Source: CAD feature listing. Evaluate the final solid. Frame: model axes, mm. A direction names the side the tool comes from. Coordinates: 2 decimals unless noted, no trailing zeros. Write each loop counter-clockwise with the first axis right and the second up, starting at its lowest first coordinate (ties: lowest second). Pieces come first, ordered by that corner, then holes. Notation, with made-up numbers: M -33.5,-38.5 L -9.5,-38.5 A20 cw -9.5,-29.5 Z; hole C 50.5,88.5 d4. An arc over 180 degrees is marked long. One line per item, written item: value. Start each with the question number.
Item 1: Cut plane D-D, the plane y = 1.4. Output: boundary loops of the cut face in (x, z) (3 decimals), then the cut area to 3 significant figures.
Item 2: Mould query, pull axis Z, two halves, no side actions, for faces 1 (the cylindrical face through (10.301, 1.521, -5.315)), 2 (the flat face through (10, 1, -15.6)), 3 (the cylindrical face through (6.031, 1.479, 1.176)). Classes: released by +Z, released by -Z, zero draft, split by the parting line, or undercut.
Item 3: Set-up query: faces 4 (the flat face through (15, 1, -5.6)), 5 (the cylindrical face through (5.067, 1.479, -12.124)). Return all of +Z, -Z, +X, -X, +Y, -Y with unobstructed straight access to the full face (end or side cutting, diameter ignored); none if empty.
Item 4: Cut plane A-A, the plane z = 2.3. Output: boundary loops of the cut face in (x, y) (3 decimals), then the cut area to 4 significant figures.
Item 5: Cut plane C-C, the plane z = -10.6. Output: boundary loops of the cut face in (x, y) (3 decimals).
Item 6: Pin query (flat end, axial travel): P1, Ø2.5, axis at x = 5, z = -10.6, coming from the -Y side; P2, Ø1.5, axis at y = 2, z = 0, coming from the +X side; P3, Ø0.9, axis at x = 15.5, y = 1, coming from the +Z side. Return the tip coordinate at first contact, or that it passes through.
Item 7: Ray query, L1, parallel to X at y = 2.3, z = -10.6 (3 decimals); L2, parallel to Z at x = 3.75, y = 1.35; L3, parallel to Z at x = 16.75, y = 0.4. Return the intervals inside material, ascending. Write a range as from..to.
Item 8: Cut plane B-B, the plane x = 5. Output: boundary loops of the cut face in (y, z) (3 decimals), then the cut area to 4 significant figures.
```python
from build123d import *

# Parameters (mm, degrees)
SKETCH1_R           = 1.525
BOSS_EXTRUDE1_DEPTH = 3
FILLET1_R           = 1


with BuildPart() as part:
    # Sketch1 → Boss-Extrude1 (new body)
    with BuildSketch(Plane(origin=(0, 0, 0), x_dir=(1, 0, 0), z_dir=(0, 1, 0))):
        Polygon((10, 5.6), (20, 5.6), (20, 15.6), (0, 15.6), (0, 0), (0, -22.6), (10, -22.6), align=None)
        with Locations(Location((5, 10.6, 0), (0, 0, 270))):
            Circle(SKETCH1_R, mode=Mode.SUBTRACT)
        with Locations(Location((15, 10.6, 0), (0, 0, 270))):
            Circle(SKETCH1_R, mode=Mode.SUBTRACT)
        with Locations(Location((5, -2.3, 0), (0, 0, 270))):
            Circle(SKETCH1_R, mode=Mode.SUBTRACT)
        with Locations(Location((5, -20.3, 0), (0, 0, 270))):
            Circle(SKETCH1_R, mode=Mode.SUBTRACT)
    extrude(amount=BOSS_EXTRUDE1_DEPTH)

    # Fillet1
    fillet1_edges = [part.edges().sort_by_distance(p)[0] for p in [
        (10, 1.5, 22.6),
        (0, 1.5, 22.6),
        (0, 1.5, -15.6),
        (20, 1.5, -15.6),
        (20, 1.5, -5.6),
        (10, 1.5, -5.6),
    ]]
    fillet(fillet1_edges, radius=FILLET1_R)


solid = part.part
```
From the geometry:
1. outline: M 0,-14.6 A1 ccw 1,-15.6 L 19,-15.6 A1 ccw 20,-14.6 L 20,-6.6 A1 ccw 19,-5.6 L 11,-5.6 A1 cw 10,-4.6 L 10,21.6 A1 ccw 9,22.6 L 1,22.6 A1 ccw 0,21.6 Z; hole C 5,-10.6 d3.05; hole C 5,2.3 d3.05; hole C 5,20.3 d3.05; hole C 15,-10.6 d3.05
1. area: 452 mm²
2. face 1: released by +Z
2. face 2: released by -Z
2. face 3: undercut
3. face 4: +Z, +X, +Y, -Y
3. face 5: +Y, -Y
4. outline: M 0,0 L 3.475,0 L 3.475,3 L 0,3 Z; M 6.525,0 L 10,0 L 10,3 L 6.525,3 Z
4. area: 20.85 mm²
5. outline: M 0,0 L 3.475,0 L 3.475,3 L 0,3 Z; M 6.525,0 L 13.475,0 L 13.475,3 L 6.525,3 Z; M 16.525,0 L 20,0 L 20,3 L 16.525,3 Z
6. P1: passes through
6. P2: stops at x = 10
6. P3: stops at z = -5.6
7. L1: x = 0..3.475, 6.525..13.475, 16.525..20
7. L2: z = -15.6..-11.47, -9.73..1.43, 3.17..19.43, 21.17..22.6
7. L3: z = -15.6..-5.6
8. outline: M 0,-15.6 L 3,-15.6 L 3,-12.125 L 0,-12.125 Z; M 0,-9.075 L 3,-9.075 L 3,0.775 L 0,0.775 Z; M 0,3.825 L 3,3.825 L 3,18.775 L 0,18.775 Z; M 0,21.825 L 3,21.825 L 3,22.6 L 0,22.6 Z
8. area: 87.15 mm²
